from build123d import *

# Parameters (mm, degrees)
BOSS_EXTRUDE1_DEPTH = 4
BOSS_EXTRUDE1_TAPER = 10
CUT_EXTRUDE1_START  = 4
SKETCH1_3_R         = 1.1
CUT_EXTRUDE1_DEPTH  = 4
CUT_EXTRUDE2_START  = 4
SKETCH1_4_R         = 8.4
SKETCH1_4_R_2       = 1.1
CUT_EXTRUDE2_DEPTH  = 3


with BuildPart() as part:
    # Sketch1 → Boss-Extrude1 (new body)
    with BuildSketch(Plane(origin=(0, 0, 0), x_dir=(1, 0, 0), z_dir=(0, 1, 0))):
        with BuildLine():
            Line((-29.672689603, -5.7), (-19.772689603, -22.847302995))
            ThreePointArc((-19.772689603, -22.847302995), (-9.9, -28.547302995), (-0.027310397, -22.847302995))
            Line((-0.027310397, -22.847302995), (9.872689603, -5.7))
            ThreePointArc((9.872689603, -5.7), (9.872689603, 5.7), (0, 11.4))
            Line((0, 11.4), (-19.8, 11.4))
            ThreePointArc((-19.8, 11.4), (-29.672689603, 5.7), (-29.672689603, -5.7))
        make_face()
    extrude(amount=BOSS_EXTRUDE1_DEPTH, taper=BOSS_EXTRUDE1_TAPER)

    # Sketch1<3> → Cut-Extrude1 (cut)
    with BuildSketch(Plane(origin=(0, 0, 0), x_dir=(1, 0, 0), z_dir=(0, 1, 0)).offset(CUT_EXTRUDE1_START)):
        with Locations(Location((-9.9, -17.147302995, 0), (0, 0, 270))):
            Circle(SKETCH1_3_R)
        with Locations(Location((0, 0, 0), (0, 0, 270))):
            Circle(SKETCH1_3_R)
        with Locations(Location((-19.8, 0, 0), (0, 0, 270))):
            Circle(SKETCH1_3_R)
    extrude(amount=-CUT_EXTRUDE1_DEPTH, mode=Mode.SUBTRACT)

    # Sketch1<4> → Cut-Extrude2 (cut)
    # profile 1 of 3: a face of its own
    with BuildSketch(Plane(origin=(0, 0, 0), x_dir=(1, 0, 0), z_dir=(0, 1, 0)).offset(CUT_EXTRUDE2_START)):
        with Locations(Location((-19.8, 0, 0), (0, 0, 270))):
            Circle(SKETCH1_4_R)
        with Locations(Location((-19.8, 0, 0), (0, 0, 270))):
            Circle(SKETCH1_4_R_2, mode=Mode.SUBTRACT)
    # profile 2 of 3: a face of its own
    with BuildSketch(Plane(origin=(0, 0, 0), x_dir=(1, 0, 0), z_dir=(0, 1, 0)).offset(CUT_EXTRUDE2_START)):
        with Locations(Location((-9.9, -17.147302995, 0), (0, 0, 270))):
            Circle(SKETCH1_4_R)
        with Locations(Location((-9.9, -17.147302995, 0), (0, 0, 270))):
            Circle(SKETCH1_4_R_2, mode=Mode.SUBTRACT)
    # profile 3 of 3: a face of its own
    with BuildSketch(Plane(origin=(0, 0, 0), x_dir=(1, 0, 0), z_dir=(0, 1, 0)).offset(CUT_EXTRUDE2_START)):
        with Locations(Location((0, 0, 0), (0, 0, 270))):
            Circle(SKETCH1_4_R)
        with Locations(Location((0, 0, 0), (0, 0, 270))):
            Circle(SKETCH1_4_R_2, mode=Mode.SUBTRACT)
    extrude(amount=-CUT_EXTRUDE2_DEPTH, mode=Mode.SUBTRACT)


solid = part.part
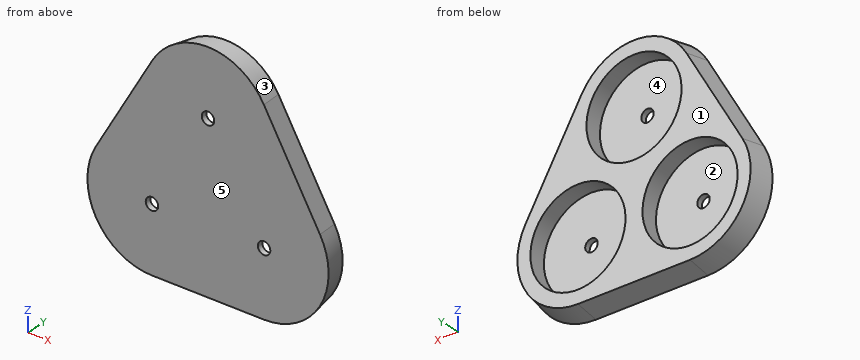
Work out the finished part from the listing and answer in its coordinate system (mm). Face numbers are marked on the shaded views. A direction names the side the tool comes from. Give positions to 0.01 mm unless a question says otherwise; leave off trailing zeros. Answer in a Markdown table with one row per item.
(1) Section A-A (z = 0) is taken. State how many separate pieces and enclosed holes the cut face has, and give its area (3 significant figures).
Results list:
| item | result |
|---|---|
| separate pieces | 3 |
| enclosed holes | 0 |
| area | 62.4 mm² |
(2) A tool of negligible diameter and unlimited length cuts with its end or side. For the marked faces 4 and 5, from which of +Z, -Z, +X, -X, +Y, -Y can it reach the whole face along a straight path? Write none if from no direction.
Results list:
| item | result |
|---|---|
| face 4 | +Y |
| face 5 | +Z, -Z, +X, -X, -Y |
(3) Flat-ended cylindrical pins translate along their axes: pin 1 Ø1 at (x, y) = (-1, 1) entering from -Z; pin 2 Ø10 at (x, z) = (-19.8, 0) entering from +Y. Find the tip coordinate at first contact, or state that the pin passes through.
Results list:
| item | result |
|---|---|
| pin 1 | stops at z = -11.31 |
| pin 2 | stops at y = 1 |
(4) Consider L1, parallel to X at y = 2.15, z = 4; L2, parallel to Z at x = -4, y = 2.5; L3, parallel to X at y = 0.35, z = 0. Determine where each line is inside the solid, lowest interval first. Write a range as [from, to].
Results list:
| item | result |
|---|---|
| L1 | x = [-30.07, -27.19], [-12.41, -7.39], [7.39, 10.27] |
| L2 | z = [-10.96, -7.39], [7.39, 11.17], [23.13, 26.38] |
| L3 | x = [-31.14, -20.9], [-18.7, -1.1], [1.1, 11.34] |
(5) For a pull along Z with two mould halves and no side action, classify the marked faces 1, 2 and 3 as pulls with the +Z half, pulls with the -Z half, needs draft (parallel to the pull), parting line crosses it, or undercut.
Results list:
| item | result |
|---|---|
| face 1 | needs draft |
| face 2 | undercut |
| face 3 | pulls with the +Z half |
